from build123d import *

# Parameters (mm, degrees)
BOSS_EXTRUDE1_DEPTH = 22.17
BOSS_EXTRUDE2_DEPTH = 9.45
CUT_EXTRUDE1_DEPTH  = 6.8
CHAMFER1_SIZE       = 0.5


with BuildPart() as part:
    # Sketch1 → Boss-Extrude1 (new body)
    with BuildSketch(Plane.XY):
        with BuildLine():
            Line((0.65, 2.275), (2.068816087, 2.275))
            ThreePointArc((2.068816087, 2.275), (3.075, 0), (2.068816087, -2.275))
            Line((2.068816087, -2.275), (-2.068816087, -2.275))
            ThreePointArc((-2.068816087, -2.275), (-3.075, 0), (-2.068816087, 2.275))
            Line((-2.068816087, 2.275), (-0.65, 2.275))
            ThreePointArc((-0.65, 2.275), (0, 2.925), (0.65, 2.275))
        make_face()
    extrude(amount=BOSS_EXTRUDE1_DEPTH)

    # Sketch2 → Boss-Extrude2 (add)
    with BuildSketch(Plane.XY.offset(22.17)):
        with BuildLine():
            ThreePointArc((-0.648810702, 5.335697674), (0, -5.375), (0.648810702, 5.335697674))
            ThreePointArc((0.648810702, 5.335697674), (0, 4.725), (-0.648810702, 5.335697674))
        make_face()
    extrude(amount=BOSS_EXTRUDE2_DEPTH)

    # Sketch3 → Cut-Extrude1 (cut)
    with BuildSketch(Plane.XY.offset(31.62)):
        with BuildLine():
            Line((-2.021756662, 2.35), (2.021756662, 2.35))
            ThreePointArc((2.021756662, 2.35), (3.1, 0), (2.021756662, -2.35))
            Line((2.021756662, -2.35), (-2.021756662, -2.35))
            ThreePointArc((-2.021756662, -2.35), (-3.1, 0), (-2.021756662, 2.35))
        make_face()
    extrude(amount=-CUT_EXTRUDE1_DEPTH, mode=Mode.SUBTRACT)

    # Chamfer1
    chamfer1_edges = [part.edges().sort_by_distance(p)[0] for p in [
        (3.075, 0, 0),
        (-3.075, 0, 0),
    ]]
    chamfer(chamfer1_edges, length=CHAMFER1_SIZE)


solid = part.part
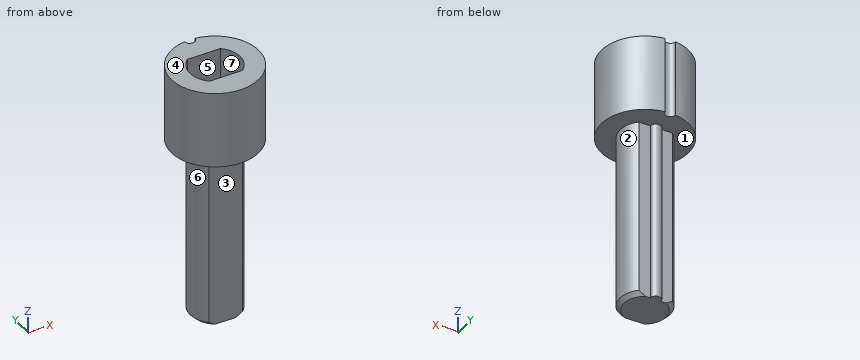
Geometry: final body of the model. Coordinates: model frame, mm. Face numbers are marked on the shaded views. A direction names the side the tool comes from. Give positions to 0.01 mm unless a question says otherwise; leave off trailing zeros. Loops run counter-clockwise (first coordinate to the right, second up) from the corner with the lowest first, then second, coordinate; pieces in that order, holes last. Notation, with made-up numbers: (72, 20.5) - (93, 20.5) arc R20 ccw to (93, 36.5) - close; hole circle Ø2 at (78.5, 87.5). An arc over 180 degrees is marked (long way). One line per question, with ' | ' between items. Start each with the question number.
(1) Reachability of the marked faces 1, 2 and 3 from +Z, -Z, +X, -X, +Y, -Y: full face, straight path, thin tool, end or side. Return the list, or none.
(2) Section query A-A on y = 0. Return loops of the section in (x, z) (3 decimals).
(3) Pull-direction query (Y, two-part tool) for the marked faces 4, 5, 6 and 7; classes: released by +Y, released by -Y, zero draft, split by the parting line, or undercut.
(4) Contact query for flat-ended pins moving along their axis: pin 1 (5 mm diameter, centred on y = 0.5, z = 9, fed in from -X) (3 decimals); pin 2 (1.1 mm diameter, centred on x = 1, z = 13, fed in from +Y); pin 3 (0.7 mm diameter, centred on x = -1.5, z = 11, fed in from +Y) (3 decimals). Output: stop coordinate, or through.
(5) Ray query, line 1 (Y direction, x = 2, z = 20.5) (3 decimals); line 2 (Z direction, x = 1.5, y = -3.75); line 3 (Y direction, x = -2, z = 27.5). Return the intervals inside material, ascending. Write a range as from..to.
(6) Section query B-B on x = 0. Return loops of the section in (y, z) (3 decimals), then the cut area to 3 significant figures.
(7) Section query C-C on z = 14. Return loops of the section in (x, y) (3 decimals).
(8) Section query D-D on y = 4.25. Return loops of the section in (x, z).
The answers:
1) face 1: -Z | face 2: -Z, +X | face 3: -Z, +X, -X, -Y
2) outline: (-5.375, 22.17) - (-3.075, 22.17) - (-3.075, 0.5) - (-2.575, 0) - (2.575, 0) - (3.075, 0.5) - (3.075, 22.17) - (5.375, 22.17) - (5.375, 31.62) - (3.1, 31.62) - (3.1, 24.82) - (-3.1, 24.82) - (-3.1, 31.62) - (-5.375, 31.62) - close
3) face 4: zero draft | face 5: undercut | face 6: split by the parting line | face 7: undercut
4) pin 1: x = -3.075 | pin 2: y = 2.74 | pin 3: y = 2.275
5) line 1: -2.275..2.275 | line 2: 22.17..31.62 | line 3: -4.99..-2.35, 2.35..4.99
6) outline: (-5.375, 22.17) - (-2.275, 22.17) - (-2.275, 0) - (2.925, 0) - (2.925, 22.17) - (4.725, 22.17) - (4.725, 31.62) - (2.35, 31.62) - (2.35, 24.82) - (-2.35, 24.82) - (-2.35, 31.62) - (-5.375, 31.62) - close | area: 179 mm2
7) outline: (-2.069, -2.275) - (2.069, -2.275) arc R3.075 ccw to (2.069, 2.275) - (0.65, 2.275) arc R0.65 ccw to (-0.65, 2.275) - (-2.069, 2.275) arc R3.075 ccw to start
8) outline: (-3.29, 22.17) - (3.29, 22.17) - (3.29, 31.62) - (-3.29, 31.62) - close
